Model file for the job. Use its own axes, mm. Face numbers are marked on the shaded views. A direction names the side the tool comes from. Round coordinates to 2 decimals unless told otherwise and drop trailing zeros. Write each loop counter-clockwise with the first axis right and the second up, starting at its lowest first coordinate (ties: lowest second). Pieces come first, ordered by that corner, then holes. Notation, with made-up numbers: (-12, -12.5) - (23, -12.5) arc R13 cw to (23, 11.5) - close; hole circle Ø2 at (34.25, 71.25). An arc over 180 degrees is marked (long way). Answer as a JSON object with one key per item and string values. Group by question number.
from build123d import *

# Parameters (mm, degrees)
F0_W     = 31.75
F0_H     = 80
F1_DEPTH = 31.75
F3_DEPTH = 31.751
F4_W     = 25.4
F4_H     = 10
F4_W_2   = 3.175
F4_H_2   = 43.2458060166
F5_DEPTH = 31.751
F6_W     = 47.7026679298
F6_H     = 12.140064659
F6_H_2   = 10.4135097936
F7_DEPTH = 31.751
F9_DEPTH = 31.751


with BuildPart() as f1:
    # F0 (on Top) → F1 (new body)
    with BuildSketch(Plane.XY):
        Rectangle(F0_W, F0_H)
    extrude(amount=F1_DEPTH)

    # F2 (on face) → F3 (cut, through all)
    with BuildSketch(Plane.YZ.offset(15.875)):
        with BuildLine():
            Line((20.065903716, 15.875), (25.065903716, 15.875))
            ThreePointArc((25.065903716, 15.875), (15.141864951, 16.7432408883), (24.7643668199, 14.1648992834))
            Line((24.7643668199, 14.1648992834), (20.065903716, 15.875))
        make_face()
        with BuildLine():
            ThreePointArc((34.9972, 11.5313441798), (32.5204583181, 14.4830099771), (29.183553277, 12.5564469533))
            ThreePointArc((29.183553277, 12.5564469533), (31.4795416819, 8.5796783824), (34.9972, 11.5313441798))
        make_face()
        with BuildLine():
            ThreePointArc((24.7643668199, 14.1648992834), (24.9899424811, 15.0067591117), (25.065903716, 15.875))
            Line((25.065903716, 15.875), (20.065903716, 15.875))
            Line((20.065903716, 15.875), (24.7643668199, 14.1648992834))
        make_face()
    extrude(amount=-F3_DEPTH, mode=Mode.SUBTRACT)

    # F4 (on face) → F5 (cut, through all)
    with BuildSketch(Plane.XY.offset(31.75)):
        with Locations((0, -45)):
            Rectangle(F4_W, F4_H)
        with Locations((14.2875, -18.3770969917)):
            Rectangle(F4_W_2, F4_H_2)
        with Locations((-14.2875, -18.3770969917)):
            Rectangle(F4_W_2, F4_H_2)
    extrude(amount=-F5_DEPTH, mode=Mode.SUBTRACT)

    # F6 (on face) → F7 (cut, through all)
    with BuildSketch(Plane.YZ.offset(15.875)):
        with Locations((-20.6055279483, 34.6450323295)):
            Rectangle(F6_W, F6_H)
        with Locations((-20.6055279483, -2.0317548968)):
            Rectangle(F6_W, F6_H_2)
    extrude(amount=-F7_DEPTH, mode=Mode.SUBTRACT)

    # F8 (on face) → F9 (cut, through all)
    with BuildSketch(Plane.XY.offset(31.75)):
        Polygon((15.875, 3.2458060166), (15.875, 40), (7.125, 40), (7.125, 11.9958060166), align=None)
    extrude(amount=-F9_DEPTH, mode=Mode.SUBTRACT)


solid = f1.part
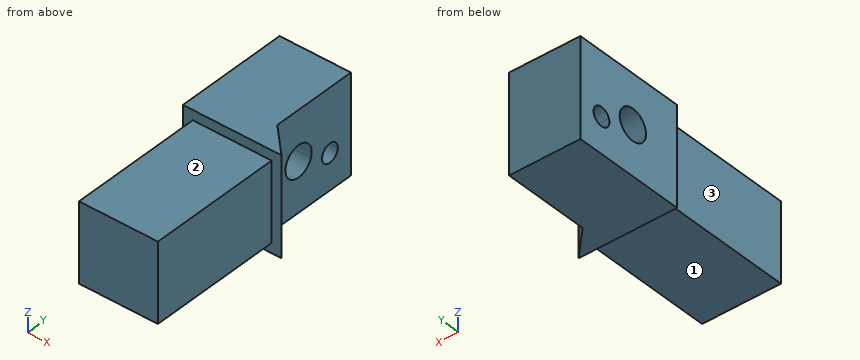
(1) Slice it at D-D (y = -2). Write the cut outline in (x, z) (3 decimals).
(2) Slice it at C-C (x = 11.5). Write the cut outline in (y, z) (3 decimals).
(3) Drill centre lines: line 1 (Z direction, x = 2, y = 20); line 2 (Z direction, x = -1, y = 32); line 3 (Y direction, x = -6.5, z = 29). Where is each one in solid material? Low to high. Write a range as from..to.
(4) Slice it at A-A (x = -7). Write the cut outline in (y, z) (3 decimals).
(5) Flat gauge pins, fed straight in: pin 1 (10 mm diameter, centred on y = -3, z = 4.5, fed in from +X); pin 2 (5 mm diameter, centred on y = -8.5, z = 16, fed in from -X); pin 3 (16 mm diameter, centred on y = 20.07, z = 15.88, fed in from +X) (3 decimals). Where does each tip first touch, or does it go through?
(6) Slice it at B-B (y = 32). Write the cut outline in (x, z) (3 decimals).
(7) 3-axis set-ups, long thin cutter, end or side, ignore diameter. For the marked faces 1, 2 and 3: which of +Z, -Z, +X, -X, +Y, -Y reach the whole face in a straight line?
Answer:
{
 "1": {"outline": "(-12.7, 3.175) - (12.7, 3.175) - (12.7, 28.575) - (-12.7, 28.575) - close"},
 "2": {"outline": "(-40, 3.175) - (3.246, 3.175) - (3.246, 0) - (7.621, 0) - (7.621, 31.75) - (3.246, 31.75) - (3.246, 28.575) - (-40, 28.575) - close"},
 "3": {"line 1": "0..10.88, 20.87..31.75", "line 2": "0..8.53, 14.53..31.75", "line 3": "3.25..40"},
 "4": {"outline": "(-40, 3.175) - (3.246, 3.175) - (3.246, 0) - (40, 0) - (40, 31.75) - (3.246, 31.75) - (3.246, 28.575) - (-40, 28.575) - close; hole circle Ø10 at (20.066, 15.875); hole circle Ø5.994 at (32, 11.531)"},
 "5": {"pin 1": "x = 12.7", "pin 2": "x = -12.7", "pin 3": "x = 7.125"},
 "6": {"outline": "(-15.875, 0) - (7.125, 0) - (7.125, 8.534) - (-15.875, 8.534) - close; (-15.875, 14.529) - (7.125, 14.529) - (7.125, 31.75) - (-15.875, 31.75) - close"},
 "7": {"face 1": "-Z, +X, -X, -Y", "face 2": "+Z, +X, -X, -Y", "face 3": "+Z, -Z, -X, -Y"}
}
